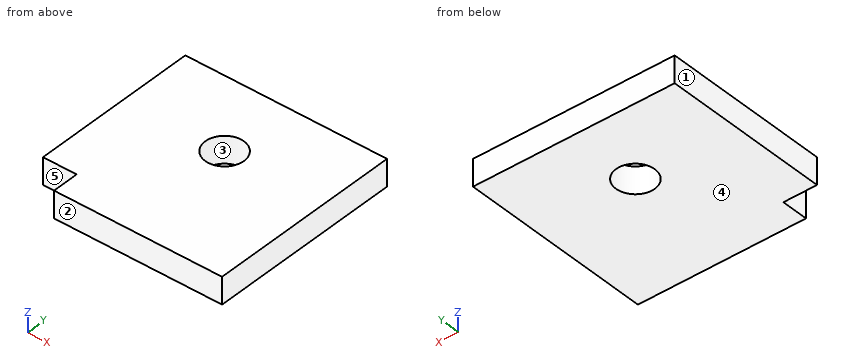
```python
from build123d import *

# Parameters (mm, degrees)
SKETCH1_R           = 2.3
BOSS_EXTRUDE1_DEPTH = 3.175


with BuildPart() as part:
    # Sketch1 → Boss-Extrude1 (new body)
    with BuildSketch(Plane.XY):
        Polygon((0, 0), (0, 20), (24, 20), (24, 0), (24, -3.175), (4, -3.175), (4, 0), align=None)
        with Locations((12, 11.35)):
            Circle(SKETCH1_R, mode=Mode.SUBTRACT)
    extrude(amount=BOSS_EXTRUDE1_DEPTH)


solid = part.part
```
For this review, take the finished solid that the model builds, in its own axes (mm). Face numbers are marked on the shaded views. A direction names the side the tool comes from. Round coordinates to 2 decimals unless told otherwise and drop trailing zeros. Write each loop counter-clockwise with the first axis right and the second up, starting at its lowest first coordinate (ties: lowest second). Pieces come first, ordered by that corner, then holes.
1) Machinability: for the marked faces 4 and 5, which of the approach directions +Z, -Z, +X, -X, +Y, -Y give a long, thin tool a straight path to every point of the face, cutting with its end or side? Answer none if there is none.
Answer below:
face 4: -Z, +X, -X, +Y, -Y
face 5: +Z, -Z, -X, -Y
2) Take a section at C-C on z = 0.85. Give the boundary of the cut face in (x, y) (3 decimals), then the cut area to 3 significant figures.
Answer below:
outline: (0, 0) - (4, 0) - (4, -3.175) - (24, -3.175) - (24, 20) - (0, 20) - close; hole circle Ø4.6 at (12, 11.35)
area: 527 mm2
3) Take a section at B-B on y = 11.35. Give the boundary of the cut face in (x, z) (3 decimals).
Answer below:
outline: (0, 0) - (9.7, 0) - (9.7, 3.175) - (0, 3.175) - close; (14.3, 0) - (24, 0) - (24, 3.175) - (14.3, 3.175) - close
4) For line 1 along Y through (x, z) = (12, 0.7) (3 decimals); line 2 along Y through (x, z) = (3.5, 0.85); line 3 along X through (y, z) = (13, 0.8), list the stretches that pass through material, from the lowest coordinate up.
Answer below:
line 1: y = -3.175 to 9.05, 13.65 to 20
line 2: y = 0 to 20
line 3: x = 0 to 10.4, 13.6 to 24
5) Insertion check: pin 1 Ø1 at (y, z) = (-1.5, 2) entering from -X. The pin has a flat end and moves straight along its axis. Give the tip position at first contact, or say it passes through.
Answer below:
pin 1: stops at x = 4
6) Mouldability with a two-part tool opening along Y and no side actions: class the marked faces 1, 2 and 3 as +Y half, -Y half, draft (parallel to the pull), parting line (faces both ways), or undercut.
Answer below:
face 1: draft
face 2: -Y half
face 3: undercut
7) Take a section at A-A on x = 12. Give the boundary of the cut face in (y, z) (3 decimals).
Answer below:
outline: (-3.175, 0) - (9.05, 0) - (9.05, 3.175) - (-3.175, 3.175) - close; (13.65, 0) - (20, 0) - (20, 3.175) - (13.65, 3.175) - close
